Work out the finished part from the listing and answer in its coordinate system (mm). A direction names the side the tool comes from. Round coordinates to 2 decimals unless told otherwise and drop trailing zeros. Write each loop counter-clockwise with the first axis right and the second up, starting at its lowest first coordinate (ties: lowest second). Pieces come first, ordered by that corner, then holes. Notation, with made-up numbers: (32, 28.5) -> (41, 28.5) arc R35 cw to (41, 61.5) -> close; hole circle Ø7 at (58, -13). An arc over 180 degrees is marked (long way). One line per item, written item: value.
```python
from build123d import *

# Parameters (mm, degrees)
SKETCH2_W           = 80
SKETCH2_H           = 80
BOSS_EXTRUDE1_DEPTH = 5
SKETCH3_R           = 2.5
SKETCH3_R_2         = 1.25
BOSS_EXTRUDE2_DEPTH = 5


with BuildPart() as part:
    # Sketch2 → Boss-Extrude1 (new body)
    with BuildSketch(Plane(origin=(0, 0, 0), x_dir=(1, 0, 0), z_dir=(0, 1, 0))):
        with Locations((40, -40)):
            Rectangle(SKETCH2_W, SKETCH2_H)
    extrude(amount=BOSS_EXTRUDE1_DEPTH)

    # Sketch3 → Boss-Extrude2 (add)
    # profile 1 of 2: a face of its own
    with BuildSketch(Plane(origin=(0, 5, 0), x_dir=(1, 0, 0), z_dir=(0, 1, 0))):
        with BuildLine():
            Line((37.5, -80), (37.5, -89.881652202))
            ThreePointArc((37.5, -89.881652202), (40, -87.381652202), (42.5, -89.881652202))
            Line((42.5, -89.881652202), (42.5, -80))
            Line((42.5, -80), (37.5, -80))
        make_face()
    # profile 2 of 2: a face of its own
    with BuildSketch(Plane(origin=(0, 5, 0), x_dir=(1, 0, 0), z_dir=(0, 1, 0))):
        with Locations((40, -89.881652202)):
            Circle(SKETCH3_R)
        with Locations(Location((40, -89.881652202, 0), (0, 0, 270))):
            Circle(SKETCH3_R_2, mode=Mode.SUBTRACT)
    extrude(amount=-BOSS_EXTRUDE2_DEPTH)


solid = part.part
```
(1) For a pull along Z with two mould halves and no side action, classify faces 4 (the face through (39, 2, 0)), 5 (the face through (39, 0, 46)), 6 (the face through (40.375, 2.535, 91.074)) as pulls with the +Z half, pulls with the -Z half, needs draft (parallel to the pull), parting line crosses it, or undercut.
Reported:
face 4: pulls with the -Z half
face 5: needs draft
face 6: undercut
(2) Flat-ended cylindrical pins translate along their axes: pin 1 Ø1 at (x, y) = (60, 4) entering from +Z; pin 2 Ø1.5 at (y, z) = (3.5, 86.5) entering from +X. Find the tip coordinate at first contact, or state that the pin passes through.
Reported:
pin 1: stops at z = 80
pin 2: stops at x = 42.5
(3) Consider probe 1 along Z at (x, y) = (58.5, 1.9). Determine where the line is inside the solid, lowest interval first.
Reported:
probe 1: z = 0 to 80
(4) A tool of negligible diameter and unlimited length cuts with its end or side. For faces 1 (the face through (37.5, 3, 85)), 2 (the face through (42.5, 3, 85)), 3 (the face through (0, 2, 41)), from which of +Z, -Z, +X, -X, +Y, -Y can it reach the whole face along a straight path? Write none if from no direction.
Reported:
face 1: +Z, -X, +Y, -Y
face 2: +Z, +X, +Y, -Y
face 3: +Z, -Z, -X, +Y, -Y
(5) Find section B-B on y = 1.5. Give the vertices of the cut face in (x, z).
Reported:
outline: (0, 0) -> (80, 0) -> (80, 80) -> (42.5, 80) -> (42.5, 89.88) arc R2.5 ccw to (37.5, 89.88) -> (37.5, 80) -> (0, 80) -> close; hole circle Ø2.5 at (40, 89.88)
(6) Find section A-A on x = 40. Give the vertices of the cut face in (y, z).
Reported:
outline: (0, 0) -> (5, 0) -> (5, 88.63) -> (0, 88.63) -> close; (0, 91.13) -> (5, 91.13) -> (5, 92.38) -> (0, 92.38) -> close
(7) Find section C-C on x = 7.5. Give the vertices of the cut face in (y, z), plus the area to 3 significant figures.
Reported:
outline: (0, 0) -> (5, 0) -> (5, 80) -> (0, 80) -> close
area: 400 mm2
